Verification items for the finished model (mm, model axes). Coordinates: 2 decimals unless noted, no trailing zeros. Write each loop counter-clockwise with the first axis right and the second up, starting at its lowest first coordinate (ties: lowest second). Pieces come first, ordered by that corner, then holes. Notation, with made-up numbers: (75, 55.25) - (113, 55.25) arc R24 cw to (113, 94.25) - close; hole circle Ø7 at (-24.75, 74.5). An arc over 180 degrees is marked (long way). Use one line per item in the form item = value. Start each with the question number.
(1) Sectioned sample at A-A (x = 0). Record the cut outline in (y, z).
(2) Sectioned sample at B-B (z = 0). Record the cut outline in (x, y), and give its area (3 significant figures).
(3) Sectioned sample at C-C (y = -292). Record the cut outline in (x, z), and give its area (3 significant figures).
(4) Material ranges on line 1 (Z direction, x = 0, y = -310); line 2 (X direction, y = -887, z = -10); line 3 (Z direction, x = -4, y = -656), recorded low to high. Write a range as [from, to].
(5) Gauge pin test, flat ends, axial feed: pin 1 Ø1 at (y, z) = (-671, -50) entering from -X; pin 2 Ø4 at (x, y) = (28.5, -503.5) entering from -Z; pin 3 Ø6 at (x, y) = (15.5, -223.5) entering from -Z. Record the tip position at first contact, or that the pin passes through.
(6) Sectioned sample at D-D (z = 131). Record the cut outline in (x, y).
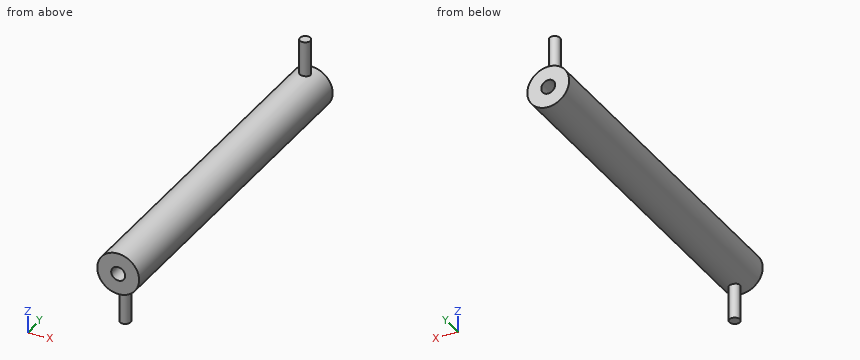
from build123d import *

# Parameters (mm, degrees)
F0_R     = 60
F2_DEPTH = 1000
F3_R     = 15
F4_DEPTH = 160
F5_R     = 15
F6_DEPTH = 160
F1_R     = 20
F7_DEPTH = 1000


with BuildPart() as f2:
    # F0 (on Front) → F2 (new body)
    with BuildSketch(Plane.XZ):
        Circle(F0_R)
    extrude(amount=F2_DEPTH)

    # F3 (on Top) → F4 (join)
    with BuildSketch(Plane.XY):
        with Locations((0, -33.885266772)):
            Circle(F3_R)
    extrude(amount=F4_DEPTH)

    # F5 (on Top) → F6 (join)
    with BuildSketch(Plane.XY):
        with Locations((0, -962.9562497139)):
            Circle(F5_R)
    extrude(amount=-F6_DEPTH)

    # F1 (on Front) → F7 (cut)
    with BuildSketch(Plane.XZ):
        Circle(F1_R)
    extrude(amount=F7_DEPTH, mode=Mode.SUBTRACT)


solid = f2.part
Answers below:
q1.outline = (-1000, -60) - (-977.96, -60) - (-977.96, -160) - (-947.96, -160) - (-947.96, -60) - (0, -60) - (0, -20) - (-1000, -20) - close; (-1000, 20) - (0, 20) - (0, 60) - (-18.89, 60) - (-18.89, 160) - (-48.89, 160) - (-48.89, 60) - (-1000, 60) - close
q2.outline = (-60, -1000) - (-20, -1000) - (-20, 0) - (-60, 0) - close; (20, -1000) - (60, -1000) - (60, 0) - (20, 0) - close
q2.area = 80,000 mm2
q3.outline = circle Ø120 at (0, 0); hole circle Ø40 at (0, 0)
q3.area = 10,100 mm2
q4.line_1 = [-60, -20], [20, 60]
q4.line_2 = [-59.16, -17.32], [17.32, 59.16]
q4.line_3 = [-59.87, -19.6], [19.6, 59.87]
q5.pin_1 = -33.91
q5.pin_2 = -53.83
q5.pin_3 = -58.68
q6.outline = circle Ø30 at (0, -33.89)
